```python
from build123d import *

# Parameters (mm, degrees)
SKETCH_1_W          = 10
SKETCH_1_H          = 10
SKETCH_1_W_2        = 8
SKETCH_1_H_2        = 8
EXTRUDE_1_DEPTH     = 26
SKETCH_2_R          = 1.5
CUT_EXTRUDE_1_DEPTH = 10
SKETCH_3_R          = 1.5
CUT_EXTRUDE_2_DEPTH = 10
SKETCH_4_R          = 3.5
CUT_EXTRUDE_3_DEPTH = 5


with BuildPart() as part:
    # 草图1 → 拉伸-薄壁1 (new body)
    with BuildSketch(Plane.XY):
        Rectangle(SKETCH_1_W, SKETCH_1_H)
        Rectangle(SKETCH_1_W_2, SKETCH_1_H_2, mode=Mode.SUBTRACT)
    extrude(amount=EXTRUDE_1_DEPTH)

    # 草图2 → 切除-拉伸1 (cut)
    with BuildSketch(Plane.ZY.offset(5)):
        with Locations((7, 0)):
            Circle(SKETCH_2_R)
        with Locations((19, 0)):
            Circle(SKETCH_2_R)
    extrude(amount=-CUT_EXTRUDE_1_DEPTH, mode=Mode.SUBTRACT)

    # 草图3 → 切除-拉伸2 (cut)
    with BuildSketch(Plane.XZ.offset(5)):
        with Locations((0, 13)):
            Circle(SKETCH_3_R)
    extrude(amount=-CUT_EXTRUDE_2_DEPTH, mode=Mode.SUBTRACT)

    # 草图4 → 切除-拉伸3 (cut)
    with BuildSketch(Plane(origin=(5, 0, 0), x_dir=(0, 0, -1), z_dir=(1, 0, 0))):
        with Locations((-19, 0)):
            Circle(SKETCH_4_R)
        with Locations((-7, 0)):
            Circle(SKETCH_4_R)
    extrude(amount=-CUT_EXTRUDE_3_DEPTH, mode=Mode.SUBTRACT)


solid = part.part
```
The listing builds one solid part. Answer for the finished solid, in the listing's coordinates (mm). A direction names the side the tool comes from. Round coordinates to 2 decimals unless told otherwise and drop trailing zeros. Order: outer loops, then holes, each group sorted by start corner. A loop starts at its lowest first (then second) coordinate and runs counter-clockwise, first axis right, second up. Notation, with made-up numbers: (12, 70.25) - (61, 70.25) arc R15 ccw to (61, 86.25) - close; hole circle Ø4 at (-27, 25.5). An arc over 180 degrees is marked (long way). Put each result on its own line as item: value. Start each with the question number.
(1) Given P1, Ø4, axis at y = 0, z = 19, coming from the +X side, flat-ended and moving along its own axis, determine where the tip first touches the part or whether it passes through.
(2) Determine the mould class of faces 1 (the flat face through (4, 0, 13)), 2 (the flat face through (-2, -4, 13)), 3 (the flat face through (-5, 0, 13)), 4 (the cylindrical face through (-4.51, 0.07, 5.5)) for opening direction X: released by +X, released by -X, zero draft, split by the parting line, or undercut.
(3) Find section D-D (y = 3). Give the vertices of the cut face in (x, z), plus the area to 3 significant figures.
(4) Find section A-A (z = 13). Give the vertices of the cut face in (x, y).
(5) Find section C-C (x = 0.25). Give the vertices of the cut face in (y, z), plus the area to 3 significant figures.
(6) Find section B-B (y = 0). Give the vertices of the cut face in (x, z), plus the area to 3 significant figures.
(7) For faces 5 (the flat face through (5, 0, 13)), 6 (the cylindrical face through (4.507, 0.154, 10.497)), 7 (the flat face through (-4, 0, 13)), determine the directions among +Z, -Z, +X, -X, +Y, -Y from which every point of the face is accessible in a straight line to the end or side of a thin tool.
(8) Straight lines are drawn through the part: probe 1 along Y at (x, z) = (-1.75, 3.25); probe 2 along Y at (x, z) = (-4.5, 7). For each, find the intervals that lie inside material, in ascending order. Write a range as from..to.
Reply:
1. P1: x = -4
2. face 1: undercut
2. face 2: undercut
2. face 3: released by -X
2. face 4: zero draft
3. outline: (-5, 0) - (-4, 0) - (-4, 26) - (-5, 26) - close; (4, 0) - (5, 0) - (5, 5.2) - (4, 5.2) - close; (4, 8.8) - (5, 8.8) - (5, 17.2) - (4, 17.2) - close; (4, 20.8) - (5, 20.8) - (5, 26) - (4, 26) - close
3. area: 44.8 mm^2
4. outline: (-5, -5) - (-1.5, -5) - (-1.5, -4) - (-4, -4) - (-4, 4) - (-1.5, 4) - (-1.5, 5) - (-5, 5) - close; (1.5, -5) - (5, -5) - (5, 5) - (1.5, 5) - (1.5, 4) - (4, 4) - (4, -4) - (1.5, -4) - close
5. outline: (-5, 0) - (-4, 0) - (-4, 11.52) - (-5, 11.52) - close; (-5, 14.48) - (-4, 14.48) - (-4, 26) - (-5, 26) - close; (4, 0) - (5, 0) - (5, 11.52) - (4, 11.52) - close; (4, 14.48) - (5, 14.48) - (5, 26) - (4, 26) - close
5. area: 46.1 mm^2
6. outline: (-5, 0) - (-4, 0) - (-4, 5.5) - (-5, 5.5) - close; (-5, 8.5) - (-4, 8.5) - (-4, 17.5) - (-5, 17.5) - close; (-5, 20.5) - (-4, 20.5) - (-4, 26) - (-5, 26) - close; (4, 0) - (5, 0) - (5, 3.5) - (4, 3.5) - close; (4, 10.5) - (5, 10.5) - (5, 15.5) - (4, 15.5) - close; (4, 22.5) - (5, 22.5) - (5, 26) - (4, 26) - close
6. area: 32.0 mm^2
7. face 5: +Z, -Z, +X, +Y, -Y
7. face 6: +X
7. face 7: +Z, -Z
8. probe 1: -5..-4, 4..5
8. probe 2: -5..-1.5, 1.5..5
